Study the drawing (mm; zero at the part's minimum x, y, z) and answer. Give positions to 0.01 mm unless a question says otherwise; leave off trailing zeros. Order: outer loops, then holes, each group sorted by start corner. A loop starts at its lowest first (then second) coordinate and runs counter-clockwise, first axis right, second up. Notation, with made-up numbers: (-22.5, 77.5) - (27.5, 77.5) arc R15 ccw to (27.5, 96.5) - close; hole circle Ø9 at (69, 26.5). An arc over 180 degrees is marked (long way). Return JSON: item names as keys, results as strings.
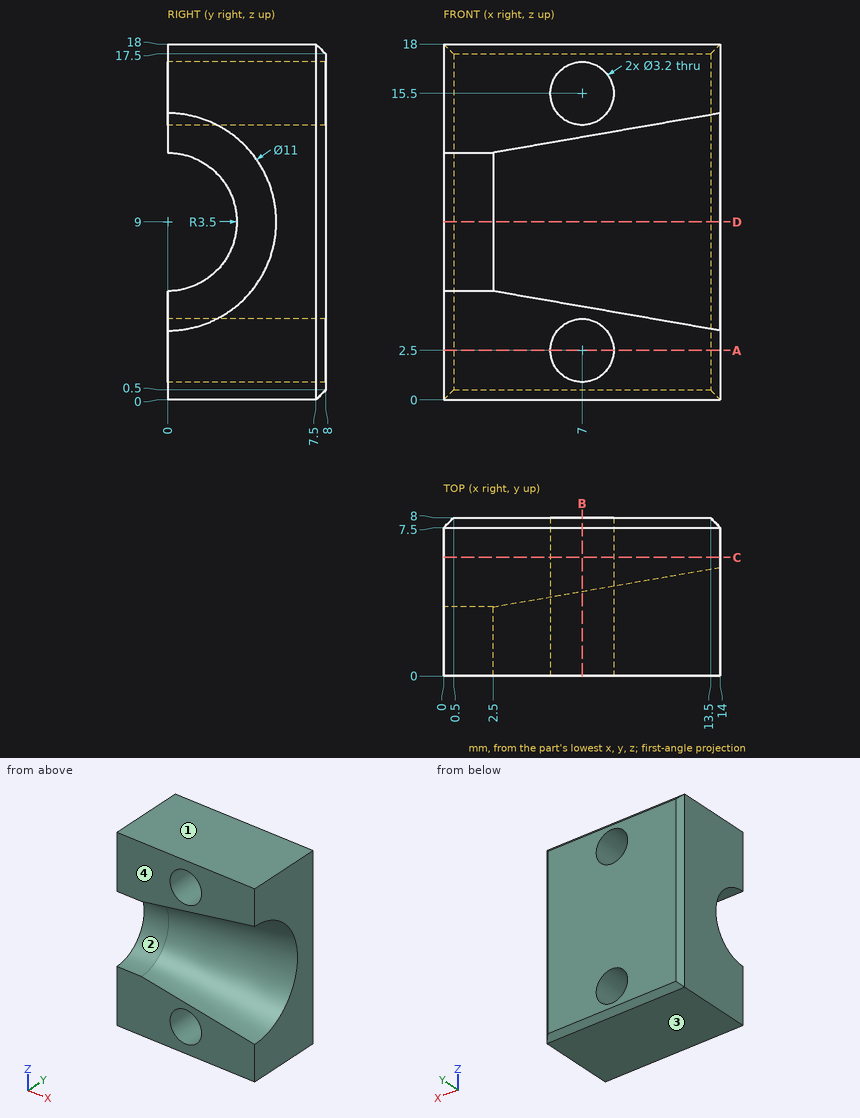
Q1. A cutting plane is placed at B-B (x = 7). Write down the section's boundary in (y, z).
Values:
{"outline": "(0, 0) - (7.5, 0) - (8, 0.5) - (8, 0.9) - (0, 0.9) - close; (0, 4.1) - (8, 4.1) - (8, 13.9) - (0, 13.9) - (0, 13.28) arc R4.28 cw to (0, 4.72) - close; (0, 17.1) - (8, 17.1) - (8, 17.5) - (7.5, 18) - (0, 18) - close"}
Q2. Given pin 1 (1.9 mm diameter, centred on x = 7, z = 2.5, fed in from -Y); pin 2 (4 mm diameter, centred on x = 8.5, z = 15.5, fed in from -Y), each flat-ended and moving along its own axis, determine where each tip first touches the part or whether it passes through.
Values:
{"pin 1": "passes through", "pin 2": "stops at y = 0"}
Q3. A cutting plane is placed at D-D (z = 9). Write down the section's boundary in (x, y).
Values:
{"outline": "(0, 3.5) - (2.5, 3.5) - (14, 5.5) - (14, 7.5) - (13.5, 8) - (0.5, 8) - (0, 7.5) - close"}
Q4. Consider L1, parallel to Z at x = 7, y = 6; L2, parallel to Z at x = 7, y = 3.25; L3, parallel to Y at x = 10, z = 11.5. Determine where each line is inside the solid, lowest interval first.
Values:
{"L1": "z = 0 to 0.9, 4.1 to 13.9, 17.1 to 18", "L2": "z = 0 to 0.9, 4.1 to 6.21, 11.79 to 13.9, 17.1 to 18", "L3": "y = 4.1 to 8"}
Q5. Determine the mould class of the marked faces 1, 2, 3 and 4 for opening direction Z: released by +Z, released by -Z, zero draft, split by the parting line, or undercut.
Values:
{"face 1": "released by +Z", "face 2": "undercut", "face 3": "released by -Z", "face 4": "zero draft"}
Q6. A cutting plane is placed at C-C (y = 6). Write down the section's boundary in (x, z).
Values:
{"outline": "(0, 0) - (14, 0) - (14, 18) - (0, 18) - close; hole circle Ø3.2 at (7, 2.5); hole circle Ø3.2 at (7, 15.5)"}
Q7. A cutting plane is placed at A-A (z = 2.5). Write down the section's boundary in (x, y).
Values:
{"outline": "(0, 0) - (5.4, 0) - (5.4, 8) - (0.5, 8) - (0, 7.5) - close; (8.6, 0) - (14, 0) - (14, 7.5) - (13.5, 8) - (8.6, 8) - close"}
